Geometry: final body of the model. Coordinates: model frame, mm. Face numbers are marked on the shaded views. A direction names the side the tool comes from. Give positions to 0.01 mm unless a question says otherwise; leave off trailing zeros. Write each loop counter-clockwise with the first axis right and the second up, starting at its lowest first coordinate (ties: lowest second). Pieces come first, ordered by that corner, then holes.
```python
from build123d import *

# Parameters (mm, degrees)
SKETCH_1_R               = 36.5
SKETCH_1_R_2             = 1.55
SKETCH_1_R_3             = 8
EXTRUDE_1_DEPTH          = 5
CUT_EXTRUDE_2_REACH      = 53.86
SKETCH_5_R               = 1.55
CUT_EXTRUDE_3_REACH      = 53.86
SKETCH_7_R               = 1.55
CUT_EXTRUDE_4_DEPTH      = 3
SKETCH_9_R               = 1.55
EXTRUDE_4_DEPTH          = 38.5
SKETCH_10_R              = 1.5
CUT_EXTRUDE_5_DEPTH      = 5
PATTERN_CIRCULAR_1_COUNT = 4
SKETCH_16_R              = 1.45
CUT_EXTRUDE_6_DEPTH      = 3
SKETCH_17_R              = 1.45
CUT_EXTRUDE_7_DEPTH      = 3
SKETCH_18_R              = 2.5
CUT_EXTRUDE_8_DEPTH      = 3


with BuildPart() as part:
    # 草图1 → 凸台-拉伸1 (new body)
    with BuildSketch(Plane(origin=(0, 0, 0), x_dir=(0, 0, -1), z_dir=(1, 0, 0))):
        Circle(SKETCH_1_R)
        with Locations((0, 12.5)):
            Circle(SKETCH_1_R_2, mode=Mode.SUBTRACT)
        with Locations((12.5, 0)):
            Circle(SKETCH_1_R_2, mode=Mode.SUBTRACT)
        with Locations((0, -12.5)):
            Circle(SKETCH_1_R_2, mode=Mode.SUBTRACT)
        with Locations((-12.5, 0)):
            Circle(SKETCH_1_R_2, mode=Mode.SUBTRACT)
        Circle(SKETCH_1_R_3, mode=Mode.SUBTRACT)
        with BuildLine():
            Line((13.594114249, 9.351473562), (22.161904167, 17.91926348))
            ThreePointArc((22.161904167, 17.91926348), (28.5, 0), (22.161904167, -17.91926348))
            Line((22.161904167, -17.91926348), (13.594114249, -9.351473562))
            ThreePointArc((13.594114249, -9.351473562), (16.5, 0), (13.594114249, 9.351473562))
        make_face(mode=Mode.SUBTRACT)
        with BuildLine():
            Line((9.351473562, 13.594114249), (17.91926348, 22.161904167))
            ThreePointArc((17.91926348, 22.161904167), (0, 28.5), (-17.91926348, 22.161904167))
            Line((-17.91926348, 22.161904167), (-9.351473562, 13.594114249))
            ThreePointArc((-9.351473562, 13.594114249), (0, 16.5), (9.351473562, 13.594114249))
        make_face(mode=Mode.SUBTRACT)
        with BuildLine():
            Line((9.351473562, -13.594114249), (17.91926348, -22.161904167))
            ThreePointArc((17.91926348, -22.161904167), (0, -28.5), (-17.91926348, -22.161904167))
            Line((-17.91926348, -22.161904167), (-9.351473562, -13.594114249))
            ThreePointArc((-9.351473562, -13.594114249), (0, -16.5), (9.351473562, -13.594114249))
        make_face(mode=Mode.SUBTRACT)
        with BuildLine():
            Line((-13.594114249, -9.351473562), (-22.161904167, -17.91926348))
            ThreePointArc((-22.161904167, -17.91926348), (-28.5, 0), (-22.161904167, 17.91926348))
            Line((-22.161904167, 17.91926348), (-13.594114249, 9.351473562))
            ThreePointArc((-13.594114249, 9.351473562), (-16.5, 0), (-13.594114249, -9.351473562))
        make_face(mode=Mode.SUBTRACT)
    extrude(amount=-EXTRUDE_1_DEPTH)

    # 草图5 → 切除-拉伸2 (cut, up to next)
    with BuildSketch(Plane(origin=(0, 0, 0), x_dir=(0, 0, -1), z_dir=(1, 0, 0)), mode=Mode.PRIVATE) as cut_extrude_2_sk1:
        with Locations((-0.006483679, -32.906479867)):
            Circle(SKETCH_5_R)
    cut_extrude_2_tool1 = extrude(cut_extrude_2_sk1.sketch, amount=-CUT_EXTRUDE_2_REACH, mode=Mode.PRIVATE) & part.part
    # 草图5 → 切除-拉伸2 (cut, up to next)
    with BuildSketch(Plane(origin=(0, 0, 0), x_dir=(0, 0, -1), z_dir=(1, 0, 0)), mode=Mode.PRIVATE) as cut_extrude_2_sk2:
        with Locations((-32.9, 0)):
            Circle(SKETCH_5_R)
    cut_extrude_2_tool2 = extrude(cut_extrude_2_sk2.sketch, amount=-CUT_EXTRUDE_2_REACH, mode=Mode.PRIVATE) & part.part
    # 草图5 → 切除-拉伸2 (cut, up to next)
    with BuildSketch(Plane(origin=(0, 0, 0), x_dir=(0, 0, -1), z_dir=(1, 0, 0)), mode=Mode.PRIVATE) as cut_extrude_2_sk3:
        with Locations((0.006479867, 32.893516321)):
            Circle(SKETCH_5_R)
    cut_extrude_2_tool3 = extrude(cut_extrude_2_sk3.sketch, amount=-CUT_EXTRUDE_2_REACH, mode=Mode.PRIVATE) & part.part
    # 草图5 → 切除-拉伸2 (cut, up to next)
    with BuildSketch(Plane(origin=(0, 0, 0), x_dir=(0, 0, -1), z_dir=(1, 0, 0)), mode=Mode.PRIVATE) as cut_extrude_2_sk4:
        with Locations((32.899996188, -0.012963547)):
            Circle(SKETCH_5_R)
    cut_extrude_2_tool4 = extrude(cut_extrude_2_sk4.sketch, amount=-CUT_EXTRUDE_2_REACH, mode=Mode.PRIVATE) & part.part
    add(cut_extrude_2_tool1.solids().sort_by_distance((0, -32.90648, 0.006484))[0], mode=Mode.SUBTRACT)
    add(cut_extrude_2_tool2.solids().sort_by_distance((0, 0, 32.9))[0], mode=Mode.SUBTRACT)
    add(cut_extrude_2_tool3.solids().sort_by_distance((0, 32.893516, -0.00648))[0], mode=Mode.SUBTRACT)
    add(cut_extrude_2_tool4.solids().sort_by_distance((0, -0.012964, -32.899996))[0], mode=Mode.SUBTRACT)

    # 草图7 → 切除-拉伸3 (cut, up to next)
    with BuildSketch(Plane(origin=(0, 0, 0), x_dir=(0, 0, -1), z_dir=(1, 0, 0)), mode=Mode.PRIVATE) as cut_extrude_3_sk1:
        with Locations((9.1971e-05, -32.90647921)):
            Circle(SKETCH_7_R)
    cut_extrude_3_tool1 = extrude(cut_extrude_3_sk1.sketch, amount=-CUT_EXTRUDE_3_REACH, mode=Mode.PRIVATE) & part.part
    add(cut_extrude_3_tool1.solids().sort_by_distance((0, -32.906479, -9.2e-05))[0], mode=Mode.SUBTRACT)

    # 草图8 → 切除-拉伸4 (cut)
    with BuildSketch(Plane(origin=(0, 0, 0), x_dir=(0, 0, -1), z_dir=(1, 0, 0))):
        Polygon((35.836823617, -1.606256173), (35.757341789, 1.738938409), (32.820577385, 3.342702418), (29.963294811, 1.601271844), (30.042776639, -1.743922738), (32.979541042, -3.347686747), align=None)
        Polygon((3.35167445, 32.972998149), (1.610243876, 35.830280724), (-1.734950706, 35.750798895), (-3.338714715, 32.814034492), (-1.597284141, 29.956751917), (1.747910441, 30.036233746), align=None)
        Polygon((-1.59971328, -35.832835914), (1.745481303, -35.753354086), (3.349245312, -32.816589682), (1.607814738, -29.959307107), (-1.737379845, -30.038788936), (-3.341143854, -32.975553339), align=None)
        Polygon((-35.826293021, 1.603700983), (-35.746811192, -1.7414936), (-32.810046789, -3.345257608), (-29.952764214, -1.603827035), (-30.032246042, 1.741367548), (-32.969010446, 3.345131557), align=None)
    extrude(amount=-CUT_EXTRUDE_4_DEPTH, mode=Mode.SUBTRACT)

    # 草图9 → 凸台-拉伸4 (add)
    # profile 1 of 4: a face of its own
    with BuildSketch(Plane.ZY.offset(5)):
        with BuildLine():
            Line((-10.975761682, 36.5), (-10.975761682, 28.456680332))
            ThreePointArc((-10.975761682, 28.456680332), (-5.582170272, 29.984819077), (0, 30.5))
            Line((0, 30.5), (0, 30.518609682))
            ThreePointArc((0, 30.518609682), (4.640042689, 30.151557641), (9.171526885, 29.088366998))
            ThreePointArc((9.171526885, 29.088366998), (10.078594454, 28.78666243), (10.975761682, 28.456680332))
            Line((10.975761682, 28.456680332), (10.975761682, 36.5))
            Line((10.975761682, 36.5), (-10.975761682, 36.5))
        make_face()
        with Locations(Location((-0.006479867, 32.893516321, 0), (0, 0, 180))):
            Circle(SKETCH_9_R, mode=Mode.SUBTRACT)
    # profile 2 of 4: a face of its own
    with BuildSketch(Plane.ZY.offset(5)):
        with BuildLine():
            Line((-29.904013109, 6), (-35.786769786, 7.180327869))
            ThreePointArc((-35.786769786, 7.180327869), (-36.5, 0), (-35.786769786, -7.180327869))
            Line((-35.786769786, -7.180327869), (-29.904013109, -6))
            ThreePointArc((-29.904013109, -6), (-30.5, 0), (-29.904013109, 6))
        make_face()
        with Locations(Location((-32.899996188, -0.012963547, 0), (0, 0, 180))):
            Circle(SKETCH_9_R, mode=Mode.SUBTRACT)
    # profile 3 of 4: a face of its own
    with BuildSketch(Plane.ZY.offset(5)):
        with BuildLine():
            Line((36.5, 10.975761682), (28.456680332, 10.975761682))
            ThreePointArc((28.456680332, 10.975761682), (30.485019718, 0.955810029), (29.088366998, -9.171526885))
            Line((29.088366998, -9.171526885), (34.810668702, -10.975761682))
            Line((34.810668702, -10.975761682), (36.5, -10.975761682))
            Line((36.5, -10.975761682), (36.5, 10.975761682))
        make_face()
        with Locations(Location((32.9, 0, 0), (0, 0, 180))):
            Circle(SKETCH_9_R, mode=Mode.SUBTRACT)
    # profile 4 of 4: a face of its own
    with BuildSketch(Plane.ZY.offset(5)):
        with BuildLine():
            Line((-6, -29.904013109), (-7.180327869, -35.786769786))
            ThreePointArc((-7.180327869, -35.786769786), (0, -36.5), (7.180327869, -35.786769786))
            Line((7.180327869, -35.786769786), (6, -29.904013109))
            ThreePointArc((6, -29.904013109), (0, -30.5), (-6, -29.904013109))
        make_face()
        with BuildLine():
            ThreePointArc((0.003040957, -34.456476044), (-1.550091963, -32.906324313), (0.003350752, -31.356483034))
            ThreePointArc((0.003350752, -31.356483034), (1.556483672, -32.906634765), (0.003040957, -34.456476044))
        make_face(mode=Mode.SUBTRACT)
    extrude(amount=EXTRUDE_4_DEPTH)

    # 草图10 → 切除-拉伸5 (cut)
    with BuildSketch(Plane(origin=(0, 0, 0), x_dir=(0, 0, -1), z_dir=(1, 0, 0))):
        with Locations((-17.5, 17.5)):
            Circle(SKETCH_10_R)
    cut_extrude_5 = extrude(amount=-CUT_EXTRUDE_5_DEPTH, mode=Mode.SUBTRACT)

    # 阵列(圆周)1: 切除-拉伸5 ×4 about axis
    pattern_circular_1_axis = Axis((0, 0, 0), (1, 0, 0))
    for i in range(1, PATTERN_CIRCULAR_1_COUNT):
        add(cut_extrude_5.rotate(pattern_circular_1_axis, i * 360 / PATTERN_CIRCULAR_1_COUNT), mode=Mode.SUBTRACT)

    # 草图16 → 切除-拉伸6 (cut)
    with BuildSketch(Plane.XY.offset(36.5)):
        with Locations((-33.875, 5.475761682)):
            Circle(SKETCH_16_R)
        with Locations((-14.625, 5.475761682)):
            Circle(SKETCH_16_R)
        with Locations((-33.875, -5.493718925)):
            Circle(SKETCH_16_R)
        with Locations((-14.625, -5.529614372)):
            Circle(SKETCH_16_R)
    extrude(amount=-CUT_EXTRUDE_6_DEPTH, mode=Mode.SUBTRACT)

    # 草图17 → 切除-拉伸7 (cut)
    with BuildSketch(Plane(origin=(0, 36.5, 0), x_dir=(1, 0, 0), z_dir=(0, 1, 0))):
        with Locations(Location((-33.875, 5.475761682, 0), (0, 0, 270))):
            Circle(SKETCH_17_R)
        with Locations(Location((-14.625, 5.475761682, 0), (0, 0, 270))):
            Circle(SKETCH_17_R)
        with Locations(Location((-33.875, -5.448898044, 0), (0, 0, 270))):
            Circle(SKETCH_17_R)
        with Locations(Location((-14.625, -5.395128045, 0), (0, 0, 270))):
            Circle(SKETCH_17_R)
    extrude(amount=-CUT_EXTRUDE_7_DEPTH, mode=Mode.SUBTRACT)

    # 草图18 → 切除-拉伸8 (cut)
    with BuildSketch(Plane(origin=(0, 0, 0), x_dir=(0, 0, -1), z_dir=(1, 0, 0))):
        with Locations((0, -12.5)):
            Circle(SKETCH_18_R)
        with Locations((12.5, 0)):
            Circle(SKETCH_18_R)
        with Locations((0, 12.5)):
            Circle(SKETCH_18_R)
        with Locations((-12.5, 0)):
            Circle(SKETCH_18_R)
    extrude(amount=-CUT_EXTRUDE_8_DEPTH, mode=Mode.SUBTRACT)


solid = part.part
```
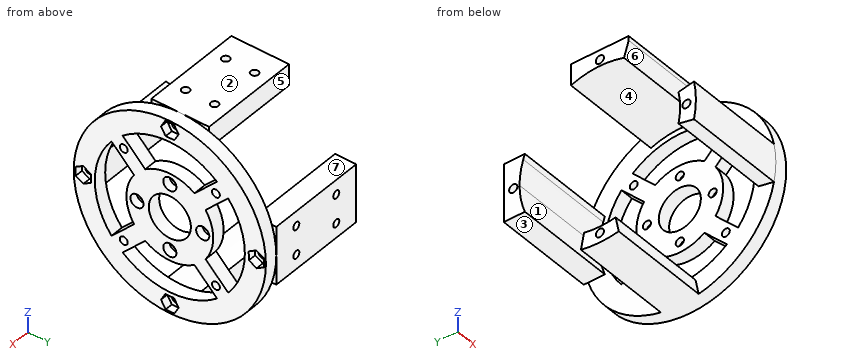
Item 1: Pin query (flat end, axial travel): pin 1 Ø2.5 at (y, z) = (-12.5, -0.5) entering from +X; pin 2 Ø1.5 at (x, z) = (-25.5, -7) entering from -Y; pin 3 Ø1.4 at (x, y) = (-15, -5.5) entering from +Z. Return the tip coordinate at first contact, or that it passes through.
Found:
pin 1: stops at x = -3
pin 2: stops at y = -35.96
pin 3: stops at z = 33.5
Item 2: Line query: L1, parallel to Z at x = -3, y = -17; L2, parallel to Z at x = -9, y = 1; L3, parallel to Z at x = -1.6, y = -17.5. Output: solid intervals per line, ascending.
Found:
L1: z = -32.3 to -22.87, -21.24 to -18.91, -16.09 to -12.76, 12.76 to 16.09, 18.91 to 21.24, 22.87 to 32.3
L2: z = -36.49 to -34.07, -31.73 to -30.48, 30.48 to 31.72, 34.08 to 36.5
L3: z = -32.03 to -22.49, -21.74 to -19, -16 to -13.26, 13.26 to 16, 19 to 21.74, 22.49 to 32.03
Item 3: Pull-direction query (Z, two-part tool) for the marked faces 4, 5, 6 and 7; classes: +Z half, -Z half, draft (parallel to the pull), parting line (faces both ways), or undercut.
Found:
face 4: undercut
face 5: draft
face 6: -Z half
face 7: +Z half
Item 4: Section B-B, the plane z = -12.5. Return the cut outline in (x, y), plus the area to 3 significant figures.
Found:
outline: (-5, -34.29) - (0, -34.29) - (0, -25.61) - (-5, -25.61) - close; (-5, -16.74) - (0, -16.74) - (0, -2.5) - (-3, -2.5) - (-3, -1.55) - (-5, -1.55) - close; (-5, 1.55) - (-3, 1.55) - (-3, 2.5) - (0, 2.5) - (0, 16.74) - (-5, 16.74) - close; (-5, 25.61) - (0, 25.61) - (0, 34.29) - (-5, 34.29) - close
area: 233 mm2
Item 5: Section A-A, the plane x = -9.5. State how many separate pieces and enclosed holes the cut face has, plus the area to 3 significant figures.
Found:
separate pieces: 4
enclosed holes: 4
area: 416 mm2
Item 6: Reachability of the marked faces 1, 2 and 3 from +Z, -Z, +X, -X, +Y, -Y: full face, straight path, thin tool, end or side. Return the list, or none.
Found:
face 1: -X
face 2: +Z, +X, -X, +Y, -Y
face 3: -Z, -X, +Y, -Y
